```python
from build123d import *

# Parameters (mm, degrees)
SKETCH9_W                      = 200
SKETCH9_H                      = 64
BASE_FLANGE2_DEPTH             = 2
EDGE_FLANGE2_STRIP_W           = 13
EDGE_FLANGE2_STRIP_H           = 2
EDGE_FLANGE2_STRIP_CUT_DEPTH   = 200
EDGE_FLANGE2_STRIP_2_W         = 13
EDGE_FLANGE2_STRIP_2_H         = 2
EDGE_FLANGE2_STRIP_CUT_2_DEPTH = 200
EDGE_FLANGE2_DEPTH             = 200
EDGE_FLANGE2_BEND_DEPTH        = 200
CUT_EXTRUDE1_DEPTH             = 143.056326857
SKETCH21_R                     = 5.5
CUT_EXTRUDE2_DEPTH             = 143.056326857
CUT_EXTRUDE3_DEPTH             = 143.056326857
SKETCH23_R                     = 7
CUT_EXTRUDE4_DEPTH             = 10


# Sheet-metal steps are written as plain solids
with BuildPart() as part:
    # Sketch9 → Base-Flange2 (new body)
    with BuildSketch(Plane(origin=(0, 0, 0), x_dir=(1, 0, 0), z_dir=(0, 1, 0))):
        Rectangle(SKETCH9_W, SKETCH9_H)
    extrude(amount=-BASE_FLANGE2_DEPTH)

    # Edge-Flange2 strip (across the edge) → Edge-Flange2 strip cut (cut)
    with BuildSketch(Plane(origin=(-100, 0, 32), x_dir=(0, 0, -1), z_dir=(1, 0, 0))):
        with Locations((-2, -1)):
            Rectangle(EDGE_FLANGE2_STRIP_W, EDGE_FLANGE2_STRIP_H)
    extrude(amount=EDGE_FLANGE2_STRIP_CUT_DEPTH, mode=Mode.SUBTRACT)

    # Edge-Flange2 strip 2 (across the edge) → Edge-Flange2 strip cut 2 (cut)
    with BuildSketch(Plane(origin=(100, 0, -32), x_dir=(0, 0, 1), z_dir=(-1, 0, 0))):
        with Locations((-2, -1)):
            Rectangle(EDGE_FLANGE2_STRIP_2_W, EDGE_FLANGE2_STRIP_2_H)
    extrude(amount=EDGE_FLANGE2_STRIP_CUT_2_DEPTH, mode=Mode.SUBTRACT)

    # Edge-Flange2 section (across the edge) → Edge-Flange2 (add)
    with BuildSketch(Plane(origin=(-100, 0, 32), x_dir=(0, 0, -1), z_dir=(1, 0, 0))):
        with BuildLine():
            Line((0, 2.5), (0, 78))
            Line((0, 78), (2, 78))
            Line((2, 78), (2, 2.5))
            ThreePointArc((2, 2.5), (2.732233047, 0.732233047), (4.5, 0))
            Line((4.5, 0), (4.5, -2))
            ThreePointArc((4.5, -2), (1.318019485, -0.681980515), (0, 2.5))
        make_face()
    extrude(amount=EDGE_FLANGE2_DEPTH)

    # Edge-Flange2 section 2 (across the edge) → Edge-Flange2 bend (add)
    with BuildSketch(Plane(origin=(100, 0, -32), x_dir=(0, 0, 1), z_dir=(-1, 0, 0))):
        with BuildLine():
            Line((0, 2.5), (0, 78))
            Line((0, 78), (2, 78))
            Line((2, 78), (2, 2.5))
            ThreePointArc((2, 2.5), (2.732233047, 0.732233047), (4.5, 0))
            Line((4.5, 0), (4.5, -2))
            ThreePointArc((4.5, -2), (1.318019485, -0.681980515), (0, 2.5))
        make_face()
    extrude(amount=EDGE_FLANGE2_BEND_DEPTH)

    # Sketch20 → Cut-Extrude1 (cut, through all)
    with BuildSketch(Plane.XY.offset(32)):
        Polygon((-100, 2.5), (-20, 78), (-100, 78), align=None)
    cut_extrude1 = extrude(amount=-CUT_EXTRUDE1_DEPTH, mode=Mode.SUBTRACT)

    # Mirror1: Cut-Extrude1 across plane
    add(cut_extrude1.mirror(Plane(origin=(0, 0, 0), x_dir=(0, 0, 1), z_dir=(1, 0, 0))), mode=Mode.SUBTRACT)

    # Sketch21 → Cut-Extrude2 (cut, through all)
    with BuildSketch(Plane.XY.offset(32)):
        with Locations((0, 66)):
            Circle(SKETCH21_R)
    extrude(amount=-CUT_EXTRUDE2_DEPTH, mode=Mode.SUBTRACT)

    # Sketch22 → Cut-Extrude3 (cut, through all)
    with BuildSketch(Plane.XY.offset(32)):
        with BuildLine():
            ThreePointArc((-11.803278689, 31.989963067), (0, 30), (11.803278689, 31.989963067))
            ThreePointArc((11.803278689, 31.989963067), (15.195977865, 38.98921962), (8.196721311, 42.381918796))
            ThreePointArc((8.196721311, 42.381918796), (0, 41), (-8.196721311, 42.381918796))
            ThreePointArc((-8.196721311, 42.381918796), (-15.195977865, 38.98921962), (-11.803278689, 31.989963067))
        make_face()
    extrude(amount=-CUT_EXTRUDE3_DEPTH, mode=Mode.SUBTRACT)

    # Sketch23 → Cut-Extrude4 (cut)
    with BuildSketch(Plane(origin=(0, 0, 0), x_dir=(1, 0, 0), z_dir=(0, 1, 0))):
        with Locations(Location((-80, 0, 0), (0, 0, 270))):
            Circle(SKETCH23_R)
        with Locations(Location((80, 0, 0), (0, 0, 270))):
            Circle(SKETCH23_R)
    extrude(amount=-CUT_EXTRUDE4_DEPTH, mode=Mode.SUBTRACT)


solid = part.part
```
Source: CAD feature listing. Evaluate the final solid. Frame: model axes, mm. A direction names the side the tool comes from. Coordinates: 2 decimals unless noted, no trailing zeros. Loops run counter-clockwise (first coordinate to the right, second up) from the corner with the lowest first, then second, coordinate; pieces in that order, holes last. Notation, with made-up numbers: M 27,29 L 77,29 A21 ccw 77,44 Z; hole C 23.25,4.5 d1. An arc over 180 degrees is marked long. Use a Markdown table: item, result. Add a question column.
Q1. Section query D-D, the plane x = 10. Return loops of the section in (y, z).
Q2. Draft query along X for faces 1 (the flat face through (-60.56, 39.72, -30.99)), 2 (the flat face through (-1, 24, 30)), 3 (the cylindrical face through (-15.155, 39.103, 31.014)), 4 (the flat face through (60.56, 39.72, 31.01)). Return one class per face: pulls with the +X half, pulls with the -X half, needs draft (parallel to the pull), parting line crosses it, or undercut.
Q3. Material intervals for L1, parallel to X at y = -1.6, z = 0; L2, parallel to Z at x = 4.5, y = 51.5; L3, parallel to Y at x = 0, z = 30.8, sorted ascending.
Q4. Section query C-C, the plane x = 80. Return loops of the section in (y, z) (3 decimals).
Q5. Access query for faces 5 (the cylindrical face through (86.94, -0.99, -0.91)), 6 (the flat face through (1, 24, -30)). Directions: +Z, -Z, +X, -X, +Y, -Y. A direction counts if a zero-diameter tool reaches every point of the face in a straight line with its end or side. Return the directions, or none.
Q6. First-contact query: pin 1 (6 mm diameter, centred on x = 62.5, z = 4, fed in from +Y). Flat tip, straight axial feed; report the tip coordinate or a pass-through.
Q7. Section query B-B, the plane y = 18. Return loops of the section in (x, z).
Q8. Section query A-A, the plane z = 0. Return loops of the section in (x, y).
Result:
| question | item | result |
|---|---|---|
| 1 | outline | M -2,-27.5 A4.5 ccw 2.5,-32 L 31.42,-32 L 31.42,-30 L 2.5,-30 A2.5 cw 0,-27.5 L 0,27.5 A2.5 cw 2.5,30 L 31.42,30 L 31.42,32 L 2.5,32 A4.5 ccw -2,27.5 Z; M 42.69,-32 L 78,-32 L 78,-30 L 42.69,-30 Z; M 42.69,30 L 78,30 L 78,32 L 42.69,32 Z |
| 2 | face 1 | pulls with the -X half |
| 2 | face 2 | needs draft |
| 2 | face 3 | undercut |
| 2 | face 4 | pulls with the +X half |
| 3 | L1 | x = -100 to -87, -73 to 73, 87 to 100 |
| 3 | L2 | z = -32 to -30, 30 to 32 |
| 3 | L3 | y = -0.56 to 30, 41 to 60.5, 71.5 to 78 |
| 4 | outline | M -2,-27.5 A4.5 ccw 2.5,-32 L 21.375,-32 L 21.375,-30 L 2.5,-30 A2.5 cw 0,-27.5 L 0,-7 L -2,-7 Z; M -2,7 L 0,7 L 0,27.5 A2.5 cw 2.5,30 L 21.375,30 L 21.375,32 L 2.5,32 A4.5 ccw -2,27.5 Z |
| 5 | face 5 | +Y, -Y |
| 5 | face 6 | +X, -X, +Y |
| 6 | pin 1 | stops at y = 0 |
| 7 | outline | M -83.58,-32 L 83.58,-32 L 83.58,-30 L -83.58,-30 Z; M -83.58,30 L 83.58,30 L 83.58,32 L -83.58,32 Z |
| 8 | outline | M -100,-2 L -87,-2 L -87,0 L -100,0 Z; M -73,-2 L 73,-2 L 73,0 L -73,0 Z; M 87,-2 L 100,-2 L 100,0 L 87,0 Z |
